Input: dimensioned drawing with shaded views. Units: mm. Origin: part minimum x, y, z. Give positions to 0.01 mm unless a question says otherwise; leave off trailing zeros. Write each loop counter-clockwise with the first axis right and the second up, starting at its lowest first coordinate (ties: lowest second). Pieces come first, ordered by that corner, then holes. Notation, with made-up numbers: (0, 65.5) -> (32, 65.5) arc R5 ccw to (32, 73.5) -> close; hole circle Ø10 at (5, 67.5). An arc over 180 degrees is marked (long way). Answer in a Markdown table with one row per item. Add a question column.
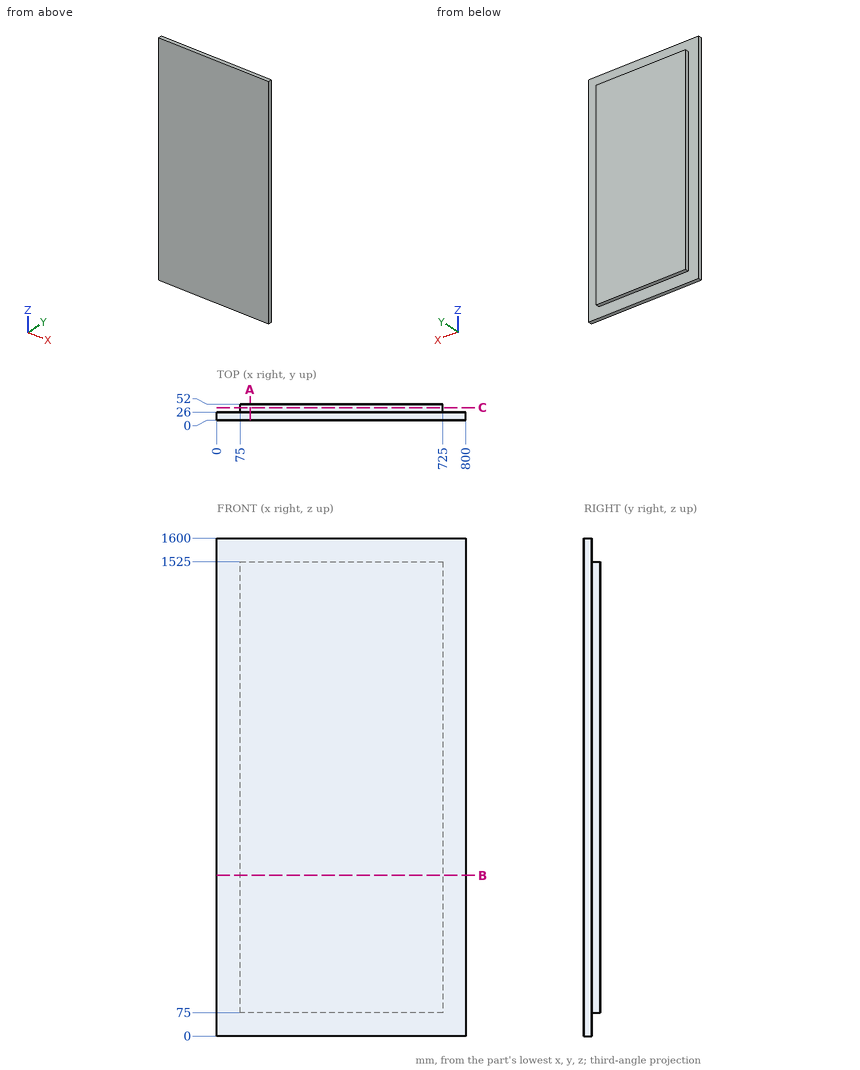
Q1. Section B-B on z = 516. Return loops of the section in (x, y), and give its area (3 significant figures).
Q2. Section C-C on y = 40.5. Return loops of the section in (x, z), and give its area (4 significant figures).
Q3. Contact query for flat-ended pins moving along their axis: pin 1 Ø1.5 at (y, z) = (42.5, 167) entering from -X; pin 2 Ø21 at (y, z) = (38, 910) entering from +X; pin 3 Ø6 at (x, y) = (132, 30.5) entering from +Z. Output: stop coordinate, or through.
Q4. Section A-A on x = 106.5. Return loops of the section in (y, z).
Q5. Line query: probe 1 along X at (y, z) = (35.5, 1472); probe 2 along Y at (x, z) = (705.5, 66); probe 3 along Z at (x, y) = (396.5, 48). Output: solid intervals per line, ascending. Write a range as from..to.
Checks:
| question | item | result |
|---|---|---|
| 1 | outline | (0, 0) -> (800, 0) -> (800, 26) -> (725, 26) -> (725, 52) -> (75, 52) -> (75, 26) -> (0, 26) -> close |
| 1 | area | 37,700 mm^2 |
| 2 | outline | (75, 75) -> (725, 75) -> (725, 1525) -> (75, 1525) -> close |
| 2 | area | 942,500 mm^2 |
| 3 | pin 1 | x = 75 |
| 3 | pin 2 | x = 725 |
| 3 | pin 3 | z = 1525 |
| 4 | outline | (0, 0) -> (26, 0) -> (26, 75) -> (52, 75) -> (52, 1525) -> (26, 1525) -> (26, 1600) -> (0, 1600) -> close |
| 5 | probe 1 | 75..725 |
| 5 | probe 2 | 0..26 |
| 5 | probe 3 | 75..1525 |
